Read the model definition and answer for the solid it produces. Units are mm, in the model's axes. A direction names the side the tool comes from. Coordinates: 2 decimals unless noted, no trailing zeros. Write each loop counter-clockwise with the first axis right and the second up, starting at its lowest first coordinate (ties: lowest second). Pieces come first, ordered by that corner, then holes. Notation, with made-up numbers: (77, 37) -> (90, 37) arc R20 cw to (90, 42) -> close; hole circle Ø9 at (52.25, 22). An arc over 180 degrees is marked (long way). Use CSV: the item, a comma, the result in double quotes.
from build123d import *

# Parameters (mm, degrees)
SKETCH2_R             = 12.5
SKETCH2_R_2           = 6.25
BOSS_EXTRUDE1_DEPTH   = 10
SKETCH2_R_3           = 21
SKETCH2_R_4           = 16
BOSS_EXTRUDE1_2_DEPTH = 10
BOSS_EXTRUDE2_DEPTH   = 6
CUT_EXTRUDE1_START    = -6
CUT_EXTRUDE1_DEPTH    = 132.802456026
CUT_EXTRUDE4_START    = 6
CUT_EXTRUDE4_DEPTH    = 132.802456026


with BuildPart() as part:
    # Sketch2 → Boss-Extrude1 (new, symmetric)
    with BuildSketch(Plane.XY):
        with Locations((0, 120)):
            Circle(SKETCH2_R)
        with Locations((0, 120)):
            Circle(SKETCH2_R_2, mode=Mode.SUBTRACT)
    extrude(amount=BOSS_EXTRUDE1_DEPTH, both=True)



with BuildPart() as body_2:
    # Sketch2 → Boss-Extrude1 2 (new, symmetric)
    with BuildSketch(Plane.XY):
        Circle(SKETCH2_R_3)
        Circle(SKETCH2_R_4, mode=Mode.SUBTRACT)
    extrude(amount=BOSS_EXTRUDE1_2_DEPTH, both=True)


with BuildPart() as part_1:
    add(part.part)

    add(body_2.part)  # Boss-Extrude2 merges body 2
    # Sketch2<3> → Boss-Extrude2 (add, symmetric)
    with BuildSketch(Plane.XY):
        with BuildLine():
            ThreePointArc((8, 110.395313644), (0, 107.5), (-8, 110.395313644))
            Line((-8, 110.395313644), (-8, 75.395313644))
            ThreePointArc((-8, 75.395313644), (-12.871500282, 40.050257874), (-20.354994984, 5.164705142))
            ThreePointArc((-20.354994984, 5.164705142), (0, 21), (20.354994984, 5.164705142))
            ThreePointArc((20.354994984, 5.164705142), (12.871500282, 40.050257874), (8, 75.395313644))
            Line((8, 75.395313644), (8, 110.395313644))
        make_face()
        with BuildLine():
            Line((-6.25, 135.825317547), (-6.25, 130.825317547))
            ThreePointArc((-6.25, 130.825317547), (0, 132.5), (6.25, 130.825317547))
            Line((6.25, 130.825317547), (6.25, 135.825317547))
            Line((6.25, 135.825317547), (-6.25, 135.825317547))
        make_face()
        with BuildLine():
            ThreePointArc((17, -12.328828006), (0, -21), (-17, -12.328828006))
            Line((-17, -12.328828006), (-17, -24.328828006))
            Line((-17, -24.328828006), (17, -24.328828006))
            Line((17, -24.328828006), (17, -12.328828006))
        make_face()
    extrude(amount=BOSS_EXTRUDE2_DEPTH, both=True)

    # Sketch4 → Cut-Extrude1 (cut, through all)
    with BuildSketch(Plane(origin=(0, 0, 0), x_dir=(0, 0, -1), z_dir=(1, 0, 0)).offset(CUT_EXTRUDE1_START)):
        with BuildLine():
            Line((4, 100), (4, 38))
            ThreePointArc((4, 38), (0, 34), (-4, 38))
            Line((-4, 38), (-4, 100))
            ThreePointArc((-4, 100), (0, 104), (4, 100))
        make_face()
    extrude(amount=-CUT_EXTRUDE1_DEPTH, mode=Mode.SUBTRACT)

    # Sketch4<4> → Cut-Extrude4 (cut, through all)
    with BuildSketch(Plane(origin=(0, 0, 0), x_dir=(0, 0, -1), z_dir=(1, 0, 0)).offset(CUT_EXTRUDE4_START)):
        with BuildLine():
            Line((4, 100), (4, 38))
            ThreePointArc((4, 38), (0, 34), (-4, 38))
            Line((-4, 38), (-4, 100))
            ThreePointArc((-4, 100), (0, 104), (4, 100))
        make_face()
    extrude(amount=CUT_EXTRUDE4_DEPTH, mode=Mode.SUBTRACT)


solid = part_1.part
1. A cutting plane is placed at A-A (z = 0). Give the vertices of the cut face in (x, y) (3 decimals), and give its area (3 significant figures).
Solutions:
outline,"(-20.355, 5.165) arc R21 ccw to (-17, -12.329) -> (-17, -24.329) -> (17, -24.329) -> (17, -12.329) arc R21 ccw to (20.355, 5.165) arc R479.998 cw to (13.976, 34) -> (6, 34) -> (6, 104) -> (8, 104) -> (8, 110.395) arc R12.5 ccw to (6.25, 130.825) -> (6.25, 135.825) -> (-6.25, 135.825) -> (-6.25, 130.825) arc R12.5 ccw to (-8, 110.395) -> (-8, 104) -> (-6, 104) -> (-6, 34) -> (-13.976, 34) arc R479.998 cw to start; hole circle Ø32 at (0, 0); hole circle Ø12.5 at (0, 120)"
area,"2,610 mm^2"
2. Find the intervals of material crossed by line 1 along Y through (x, z) = (0, 5); line 2 along Z through (x, y) = (-7.5, 58.5); line 3 along Y through (x, z) = (-8, -6.25), in increasing order.
Solutions:
line 1,"y = -24.33 to -16, 16 to 113.75, 126.25 to 135.83"
line 2,"z = -6 to -4, 4 to 6"
line 3,"y = -19.42 to -13.86, 13.86 to 19.42, 110.4 to 129.6"
3. For a pull along Z with two mould halves and no side action, classify faces 4 (the flat face through (8, 63, -4)), 5 (the flat face through (0, 59, -6)), 6 (the flat face through (-6, 117, 10)), 7 (the flat face through (6.25, 133, 0)) as pulls with the +Z half, pulls with the -Z half, needs draft (parallel to the pull), parting line crosses it, or undercut.
Solutions:
face 4,"undercut"
face 5,"pulls with the -Z half"
face 6,"pulls with the +Z half"
face 7,"needs draft"
4. A cutting plane is placed at D-D (y = 56.5). Give the vertices of the cut face in (x, z).
Solutions:
outline,"(-10.27, -6) -> (10.27, -6) -> (10.27, -4) -> (6, -4) -> (6, 4) -> (10.27, 4) -> (10.27, 6) -> (-10.27, 6) -> (-10.27, 4) -> (-6, 4) -> (-6, -4) -> (-10.27, -4) -> close"
5. A cutting plane is placed at B-B (y = 0). Give the vertices of the cut face in (x, z).
Solutions:
outline,"(-21, -10) -> (-16, -10) -> (-16, 10) -> (-21, 10) -> close; (16, -10) -> (21, -10) -> (21, 10) -> (16, 10) -> close"
6. Each of these flat-tipped pins is pushed along its axis until it touches: pin 1 Ø1 at (x, y) = (15.5, 16) entering from +Z; pin 2 Ø12 at (y, z) = (1, -3) entering from +X; pin 3 Ø3 at (y, z) = (73, 0.5) entering from +X; pin 4 Ø3 at (x, y) = (2, 102) entering from -Z. Where does it stop, or does it pass through?
Solutions:
pin 1,"stops at z = 6"
pin 2,"stops at x = 21"
pin 3,"stops at x = 6"
pin 4,"stops at z = -6"
7. A cutting plane is placed at C-C (x = 0). Give the vertices of the cut face in (y, z).
Solutions:
outline,"(-24.33, -6) -> (-21, -6) -> (-21, -10) -> (-16, -10) -> (-16, 10) -> (-21, 10) -> (-21, 6) -> (-24.33, 6) -> close; (16, -10) -> (21, -10) -> (21, -6) -> (107.5, -6) -> (107.5, -10) -> (113.75, -10) -> (113.75, 10) -> (107.5, 10) -> (107.5, 6) -> (21, 6) -> (21, 10) -> (16, 10) -> close; (126.25, -10) -> (132.5, -10) -> (132.5, -6) -> (135.83, -6) -> (135.83, 6) -> (132.5, 6) -> (132.5, 10) -> (126.25, 10) -> close"
8. A tool of negligible diameter and unlimited length cuts with its end or side. For faces 1 (the flat face through (0, -22, 6)), 2 (the cylindrical face through (-7, 104, 0)), 3 (the cylindrical face through (-14.216, 32.742, -0.084)), from which of +Z, -Z, +X, -X, +Y, -Y can it reach the whole face along a straight path? Write none if from no direction.
Solutions:
face 1,"+Z, -Y"
face 2,"-X"
face 3,"+Z, -Z, -X"
